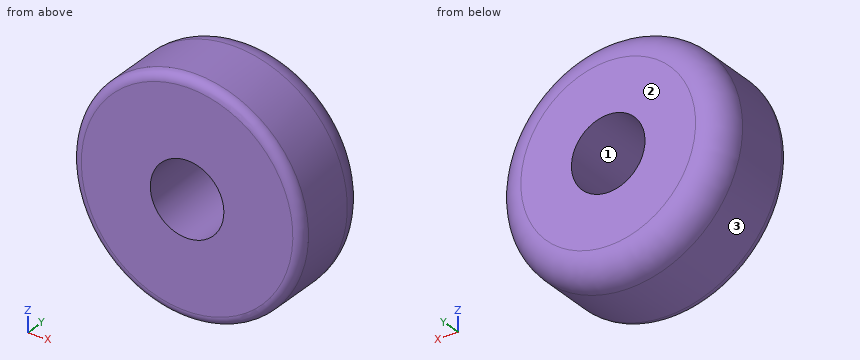
from build123d import *

# Parameters (mm, degrees)
SKETCH1_R           = 12.5
BOSS_EXTRUDE1_DEPTH = 10
FILLET1_R           = 3
SKETCH2_R           = 4
CUT_EXTRUDE1_DEPTH  = 21.310096012
FILLET2_R           = 1


with BuildPart() as part:
    # Sketch1 → Boss-Extrude1 (new body)
    with BuildSketch(Plane(origin=(0, 0, 0), x_dir=(1, 0, 0), z_dir=(0, 1, 0))):
        with Locations(Location((0, 0, 0), (0, 0, 270))):
            Circle(SKETCH1_R)
    extrude(amount=BOSS_EXTRUDE1_DEPTH)

    # Fillet1
    fillet1_edges = [part.edges().sort_by_distance(p)[0] for p in [
        (0, 10, -12.5),
    ]]
    fillet(fillet1_edges, radius=FILLET1_R)

    # Sketch2 → Cut-Extrude1 (cut, through all)
    with BuildSketch(Plane(origin=(0, 10, 0), x_dir=(1, 0, 0), z_dir=(0, 1, 0))):
        with Locations(Location((0, 0, 0), (0, 0, 270))):
            Circle(SKETCH2_R)
    extrude(amount=-CUT_EXTRUDE1_DEPTH, mode=Mode.SUBTRACT)

    # Fillet2
    fillet2_edges = [part.edges().sort_by_distance(p)[0] for p in [
        (0, 0, -12.5),
    ]]
    fillet(fillet2_edges, radius=FILLET2_R)


solid = part.part
For this review, take the finished solid that the model builds, in its own axes (mm). Face numbers are marked on the shaded views. Coordinates: 2 decimals unless noted, no trailing zeros. Order: outer loops, then holes, each group sorted by start corner. A loop starts at its lowest first (then second) coordinate and runs counter-clockwise, first axis right, second up. Notation, with made-up numbers: (87.25, 76.5) - (105.25, 76.5) arc R8 cw to (105.25, 84.5) - close; hole circle Ø6 at (35, 68). An arc over 180 degrees is marked (long way). Use one line per item in the form item = value.
Q1. For probe 1 along X at (y, z) = (5, 0); probe 2 along X at (y, z) = (8, 0); probe 3 along Y at (x, z) = (8.25, -5), list the stretches that pass through material, from the lowest coordinate up. Write a range as from..to.
Checked values:
probe_1 = -12.5..-4, 4..12.5
probe_2 = -12.33..-4, 4..12.33
probe_3 = 0..10
Q2. Consider section A-A (z = 0). Give the boundary of the cut face in (x, y), then the cut area to 3 significant figures.
Checked values:
outline = (-12.5, 1) arc R1 ccw to (-11.5, 0) - (-4, 0) - (-4, 10) - (-9.5, 10) arc R3 ccw to (-12.5, 7) - close; (4, 0) - (11.5, 0) arc R1 ccw to (12.5, 1) - (12.5, 7) arc R3 ccw to (9.5, 10) - (4, 10) - close
area = 166 mm2
Q3. Draft analysis for pull direction Z (two halves, no side actions). For the marked faces 1, 2 and 3, state which applies: +Z half, -Z half, draft (parallel to the pull), parting line (faces both ways), or undercut.
Checked values:
face_1 = undercut
face_2 = draft
face_3 = parting line
Q4. Consider section B-B (y = 4.25). Give the boundary of the cut face in (x, z).
Checked values:
outline = circle Ø25 at (0, 0); hole circle Ø8 at (0, 0)
Q5. For P1, Ø2, axis at y = 3, z = -9.5, coming from the -X side; P2, Ø4, axis at x = 4.5, y = 5, coming from the -Z side, all flat-tipped, find the tip position at first contact; note any pin that passes through.
Checked values:
P1 = -9.17
P2 = -12.25
Q6. Consider section C-C (y = 8.75). Give the boundary of the cut face in (x, z).
Checked values:
outline = circle Ø23.87 at (0, 0); hole circle Ø8 at (0, 0)
